Source: three-view drawing plus pictorial views. Frame: mm from the lowest corner of the part. Coordinates: 2 decimals unless noted, no trailing zeros. Order: outer loops, then holes, each group sorted by start corner. A loop starts at its lowest first (then second) coordinate and runs counter-clockwise, first axis right, second up. Notation, with made-up numbers: (60.25, 16) -> (115.25, 16) arc R35 ccw to (115.25, 49) -> close; hole circle Ø10 at (36, 53.5). An arc over 180 degrees is marked (long way). Use one line per item in the form item = value. Start each with the question number.
1) Ray query, line 1 along Z through (x, y) = (208, 527); line 2 along Y through (x, z) = (253, 199). Return the intervals inside material, ascending.
2) Pin query (flat end, axial travel): pin 1 (16 mm diameter, centred on x = 195, z = 102, fed in from +Y); pin 2 (22 mm diameter, centred on x = 296, y = 7.5, fed in from -Z); pin 3 (10 mm diameter, centred on y = 487.5, z = 199, fed in from -X). Return the tip coordinate at first contact, or that it passes through.
3) Section query A-A on x = 356. Output: boundary loops of the cut face in (y, z).
4) Section query B-B on y = 636. Output: boundary loops of the cut face in (x, z), then the cut area to 3 significant figures.
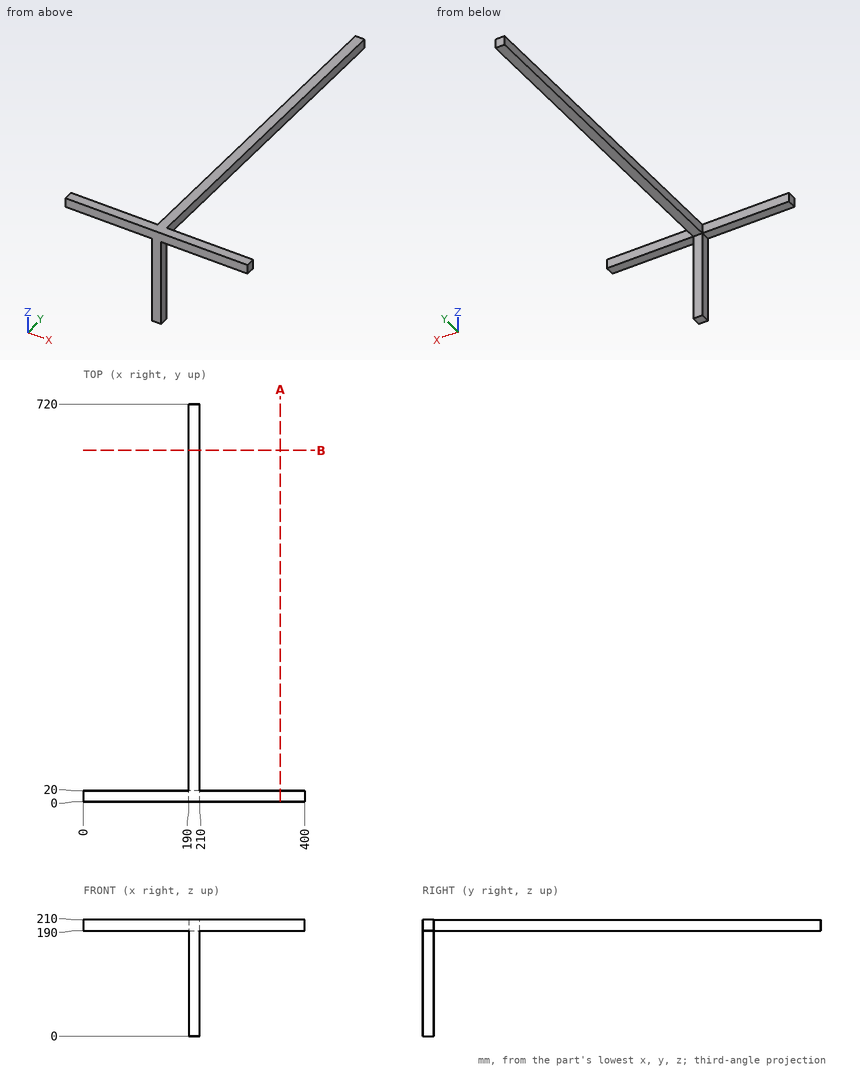
Answers below:
q1.line_1 = 190 to 210
q1.line_2 = 0 to 20
q2.pin_1 = 20
q2.pin_2 = 190
q2.pin_3 = 190
q3.outline = (0, 190) -> (20, 190) -> (20, 210) -> (0, 210) -> close
q4.outline = (190, 190) -> (210, 190) -> (210, 210) -> (190, 210) -> close
q4.area = 400 mm^2
